from build123d import *

# Parameters (mm, degrees)
F1_DEPTH = 194.5
F2_DEPTH = 194.5
F3_R     = 15
F5_R     = 100


with BuildPart() as f1:
    # F0 (on Top) → F1 (new body)
    with BuildSketch(Plane.XY):
        Polygon((-1043.9980842894, 48), (0, 50), (0, 244.1787458936), (-201.2003287221, 338), (-1043.9980842894, 338), (-1043.9980842894, 50), align=None)
    extrude(amount=F1_DEPTH)

    # F0 (on Top) → F2 (join)
    with BuildSketch(Plane.XY):
        Polygon((-1043.9980842894, 48), (0, 50), (0, 244.1787458936), (-201.2003287221, 338), (-1043.9980842894, 338), (-1043.9980842894, 50), align=None)
    extrude(amount=-F2_DEPTH)

    # F3 (on Front) → F4 (join, up to the next surface of F1)
    with BuildSketch(Plane.XZ):
        with Locations((-843, 163.5)):
            Circle(F3_R)
        with Locations((-843, -163.5)):
            Circle(F3_R)
        with Locations((-372, 163.5)):
            Circle(F3_R)
        with Locations((-372, -163.5)):
            Circle(F3_R)
    extrude(until=Until.NEXT, dir=(0, 1, 0))

    # F5
    f5_edges = [f1.edges().sort_by_distance(p)[0] for p in [
        (-1043.998084, 338, 0),
        (-1043.998084, 193, 194.5),
        (-1043.998084, 48, 0),
        (-1043.998084, 193, -194.5),
    ]]
    fillet(f5_edges, radius=F5_R)


solid = f1.part
Can you work these out from the model? Positions are in its coordinate system, mm. A direction names the side the tool comes from. Give positions to 0.01 mm unless a question says otherwise; leave off trailing zeros. Loops run counter-clockwise (first coordinate to the right, second up) from the corner with the lowest first, then second, coordinate; pieces in that order, holes last. Notation, with made-up numbers: M 50.5,41.5 L 68.5,41.5 A22 ccw 68.5,76.5 Z; hole C 29,5 d2. An arc over 180 degrees is marked long. One line per item, written item: value. Start each with the question number.
1) On a 3-axis mill with a long thin cutter (end or side, diameter ignored), from which of +Z, -Z, +X, -X, +Y, -Y can I reach the whole of each face in a straight line? I mean faces 1 (the face through (-479, 195, 194.5)), 2 (the face through (-829.144, 23.868, -169.245)). Say none if no direction works.
2) If we section it at A-A, the plane z = -67: Write out the boundary of the cut face in (x, y).
3) If I drill on line 1 (Y direction, x = -410, z = -151); line 2 (Y direction, x = -800, z = -129); line 3 (X direction, y = 37, z = 174), over which ranges is the centre line in solid material (lowest first)? Write a range as [from, to].
4) If we section it at D-D, the plane z = -163.5: Write out the boundary of the cut face in (x, y), and give its area (3 significant figures).
5) If we section it at B-B, the plane x = -372: Write out the boundary of the cut face in (y, z), and give its area (3 significant figures).
6) I'm going to push flat-ended pins straight in: pin 1 (2 mm diameter, centred on y = 93.5, z = 118, fed in from -X); pin 2 (3 mm diameter, centred on x = -909, z = 132.5, fed in from -Y). Where does each tip first touch, or does it pass through?
7) Thinking about a two-plate mould opening in X: for faces 3 (the face through (-1043.998, 194, 1)), 4 (the face through (-829.144, 23.868, 157.755)), 5 (the face through (-372, 0, -163)), which applies, +X half, -X half, draft (parallel to the pull), parting line (faces both ways), or undercut?
8) If we section it at C-C, the plane y = 89: Write out the boundary of the cut face in (x, z), and give its area (3 significant figures).
Completed:
1. face 1: +Z, +X, -X, +Y, -Y
1. face 2: -Y
2. outline: M -1044,148.19 A100 ccw -943.81,48.19 L 0,50 L 0,244.18 L -201.2,338 L -944,338 A100 ccw -1044,238 Z
3. line 1: y = [49.21, 338]
3. line 2: y = [48.47, 338]
3. line 3: x = [-853.71, -832.29], [-382.71, -361.29]
4. outline: M -1016.38,79.19 A100 ccw -943.81,48.19 L -858,48.36 L -858,0 L -828,0 L -828,48.41 L -387,49.26 L -387,0 L -357,0 L -357,49.32 L 0,50 L 0,244.18 L -201.2,338 L -944,338 A100 ccw -1016.38,307 Z
4. area: 286,000 mm^2
5. outline: M 0,-178.5 L 49.29,-178.5 L 49.29,-194.5 L 338,-194.5 L 338,194.5 L 49.29,194.5 L 49.29,178.5 L 0,178.5 L 0,148.5 L 49.29,148.5 L 49.29,-148.5 L 0,-148.5 Z
5. area: 115,000 mm^2
6. pin 1: stops at x = -1028.36
6. pin 2: stops at y = 48.26
7. face 3: -X half
7. face 4: undercut
7. face 5: draft
8. outline: M -1024.6,-153.69 A100 ccw -944,-194.5 L 0,-194.5 L 0,194.5 L -944,194.5 A100 ccw -1024.6,153.69 Z
8. area: 397,000 mm^2
